Part model, mm, in its own coordinate system. A direction names the side the tool comes from. Coordinates: 2 decimals unless noted, no trailing zeros. Write each loop counter-clockwise with the first axis right and the second up, starting at its lowest first coordinate (ties: lowest second). Pieces come first, ordered by that corner, then holes. Notation, with made-up numbers: (-29, -9) - (16, -9) arc R21 cw to (16, 2) - close; hole circle Ø4 at (31, 8.5). An arc over 180 degrees is marked (long way). Use a Markdown table: item, result.
```python
from build123d import *

# Parameters (mm, degrees)
BOSS_EXTRUDE1_DEPTH = 13.525
SKETCH3_W           = 11.025
SKETCH3_H           = 14.2
CUT_EXTRUDE1_DEPTH  = 5
SKETCH4_R           = 2
BOSS_PIVOT_DEPTH    = 1
BOSS_PIVOT_TAPER    = 15
SKETCH6_R           = 2.1
PIVOT_RECESS_DEPTH  = 1.25
PIVOT_RECESS_TAPER  = 15
CHAMFER5_SIZE       = 5
FILLET2_R           = 5
FILLET3_R           = 2.5
SKETCH8_W           = 3.997196271
SKETCH8_H           = 14.2
BOSS_EXTRUDE4_DEPTH = 1.25
FILLET4_R           = 1


with BuildPart() as part:
    # Sketch1 → Boss-Extrude1 (new body)
    with BuildSketch(Plane.XY):
        Polygon((5.35, 3.25), (5.35, 1.25), (-4.5, 1.25), (-4.5, 0), (8.05, 0), (8.05, 1.5), (17.2, 1.5), (17.2, 2.75), (9.35, 2.75), (9.35, 16.95), (17.2, 16.95), (17.2, 18.2), (8.05, 18.2), (8.05, 19.7), (-4.5, 19.7), (-4.5, 18.45), (5.35, 18.45), align=None)
    extrude(amount=BOSS_EXTRUDE1_DEPTH)

    # Sketch3 → Cut-Extrude1 (cut)
    with BuildSketch(Plane(origin=(9.35, 0, 0), x_dir=(0, 0, -1), z_dir=(1, 0, 0))):
        with Locations((-6.7625, 9.85)):
            Rectangle(SKETCH3_W, SKETCH3_H)
    extrude(amount=-CUT_EXTRUDE1_DEPTH, mode=Mode.SUBTRACT)

    # Sketch4 → boss pivot (add)
    with BuildSketch(Plane.XZ.offset(-18.45)):
        with Locations((0, 6.7625)):
            Circle(SKETCH4_R)
    boss_pivot = extrude(amount=BOSS_PIVOT_DEPTH, taper=BOSS_PIVOT_TAPER)

    # Sketch6 → pivot recess (cut)
    with BuildSketch(Plane(origin=(0, 18.2, 0), x_dir=(1, 0, 0), z_dir=(0, 1, 0))):
        with Locations((12.7, -6.7625)):
            Circle(SKETCH6_R)
    pivot_recess = extrude(amount=-PIVOT_RECESS_DEPTH, taper=PIVOT_RECESS_TAPER, mode=Mode.SUBTRACT)

    # Mirror1: boss pivot, pivot recess across plane
    add(boss_pivot.mirror(Plane.ZX.offset(9.85)))
    add(pivot_recess.mirror(Plane.ZX.offset(9.85)), mode=Mode.SUBTRACT)

    # Chamfer5
    chamfer5_edges = [part.edges().sort_by_distance(p)[0] for p in [
        (-4.5, 0.625, 0),
        (-4.5, 19.075, 0),
        (17.2, 17.575, 0),
        (17.2, 2.125, 0),
    ]]
    chamfer(chamfer5_edges, length=CHAMFER5_SIZE)

    # Fillet2
    fillet2_edges = [part.edges().sort_by_distance(p)[0] for p in [
        (17.2, 17.575, 5),
        (17.2, 2.125, 5),
        (-4.5, 0.625, 5),
        (-4.5, 19.075, 5),
    ]]
    fillet(fillet2_edges, radius=FILLET2_R)

    # Fillet3
    fillet3_edges = [part.edges().sort_by_distance(p)[0] for p in [
        (0.5, 19.075, 0),
        (0.5, 0.625, 0),
        (12.2, 2.125, 0),
        (12.2, 17.575, 0),
    ]]
    fillet(fillet3_edges, radius=FILLET3_R)

    # Sketch8 → Boss-Extrude4 (add)
    with BuildSketch(Plane.XY.offset(13.525)):
        with Locations((10.933634912, 9.85)):
            Rectangle(SKETCH8_W, SKETCH8_H)
    extrude(amount=-BOSS_EXTRUDE4_DEPTH)

    # Fillet4
    fillet4_edges = [part.edges().sort_by_distance(p)[0] for p in [
        (12.932233047, 16.95, 12.9),
        (12.932233047, 2.75, 12.9),
    ]]
    fillet(fillet4_edges, radius=FILLET4_R)


solid = part.part
```
Item 1: Which spindle directions (+Z, -Z, +X, -X, +Y, -Y) get a long thin tool onto all of the face, cutting with end or side? Do faces 5 (the face through (7, 10, 1.25)), 6 (the face through (8.05, 1, 7)), 7 (the face through (0, 2.25, 7)). Say none if no direction does.
From the geometry:
| item | result |
|---|---|
| face 5 | +X, -X |
| face 6 | +Z, -Z, +X, -Y |
| face 7 | +Z, -Z, -X |
Item 2: Drill centre lines: probe 1 along Y at (x, z) = (5.5, 7.5); probe 2 along Y at (x, z) = (3, 10.25); probe 3 along X at (y, z) = (16, 1). Where is each one in solid material? Low to high.
From the geometry:
| item | result |
|---|---|
| probe 1 | 0 to 2.75, 16.95 to 19.7 |
| probe 2 | 0 to 1.25, 18.45 to 19.7 |
| probe 3 | 5.35 to 9.35 |
Item 3: Band-saw the part on B-B, the plane y = 14.25. Give the cut face in (x, z) (3 decimals), then the cut area to 3 significant figures.
From the geometry:
| item | result |
|---|---|
| outline | (5.35, 0) - (9.35, 0) - (9.35, 1.25) - (5.35, 1.25) - close; (5.35, 12.275) - (12.932, 12.275) - (12.932, 13.525) - (5.35, 13.525) - close |
| area | 14.5 mm^2 |
Item 4: Drop flat-ended pins along their axis: P1, Ø1, axis at x = 0.5, y = 15.5, coming from the +Z side; P2, Ø1, axis at x = 10.5, z = 10.5, coming from the +Y side; P3, Ø1.4, axis at y = 12.5, z = 13, coming from the +X side; P4, Ø4, axis at y = 3, z = 4.5, coming from the +X side. Give the stop position or say it passes through.
From the geometry:
| item | result |
|---|---|
| P1 | through |
| P2 | y = 18.2 |
| P3 | x = 12.93 |
| P4 | x = 17.17 |
Item 5: Two-plate mould, pull along X, no slides. Class faces 1 (the face through (10.883, 2.55, 6.683)), 2 (the face through (12.108, 17.584, 0.185)), 3 (the face through (-4.5, 1, 10)), 4 (the face through (2, 1.25, 8)): pulls with the +X half, pulls with the -X half, needs draft (parallel to the pull), parting line crosses it, or undercut.
From the geometry:
| item | result |
|---|---|
| face 1 | undercut |
| face 2 | pulls with the +X half |
| face 3 | pulls with the -X half |
| face 4 | undercut |
Item 6: Band-saw the part on C-C, the plane z = 10.5. Give the cut face in (x, y), then the cut area to 4 significant figures.
From the geometry:
| item | result |
|---|---|
| outline | (-4.5, 0) - (8.05, 0) - (8.05, 1.5) - (17.2, 1.5) - (17.2, 2.75) - (5.35, 2.75) - (5.35, 1.25) - (-4.5, 1.25) - close; (-4.5, 18.45) - (5.35, 18.45) - (5.35, 16.95) - (17.2, 16.95) - (17.2, 18.2) - (8.05, 18.2) - (8.05, 19.7) - (-4.5, 19.7) - close |
| area | 62.35 mm^2 |
Item 7: Band-saw the part on A-A, the plane z = 3.25. Give the cut face in (x, y).
From the geometry:
| item | result |
|---|---|
| outline | (-2.75, 0) - (8.05, 0) - (8.05, 1.5) - (15.45, 1.5) - (15.45, 2.75) - (5.35, 2.75) - (5.35, 1.25) - (-2.75, 1.25) - close; (-2.75, 18.45) - (5.35, 18.45) - (5.35, 16.95) - (15.45, 16.95) - (15.45, 18.2) - (8.05, 18.2) - (8.05, 19.7) - (-2.75, 19.7) - close |
Item 8: Band-saw the part on D-D, the plane y = 16.25. Give the cut face in (x, z) (3 decimals), then the cut area to 3 significant figures.
From the geometry:
| item | result |
|---|---|
| outline | (5.35, 0) - (9.35, 0) - (9.35, 1.25) - (5.35, 1.25) - close; (5.35, 12.275) - (12.978, 12.275) - (12.978, 13.525) - (5.35, 13.525) - close |
| area | 14.5 mm^2 |
